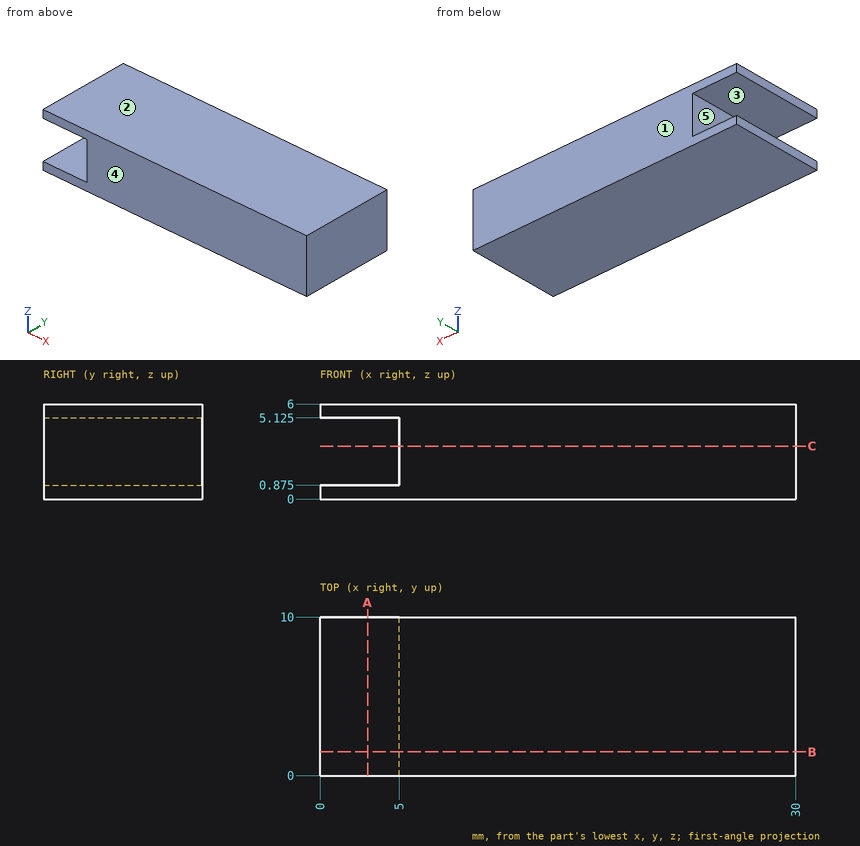
Answer from the drawing. Dimensions are ordinates in mm from the lowest x, y and z of the part. A direction names the side the tool comes from. Coordinates: 2 decimals unless noted, no trailing zeros. Order: outer loops, then holes, each group sorted by start corner. A loop starts at its lowest first (then second) coordinate and runs counter-clockwise, first axis right, second up. Notation, with made-up numbers: (-31.5, 34) - (-19.5, 34) arc R12 cw to (-19.5, 38) - close; hole circle Ø3 at (-14, 87). An arc over 180 degrees is marked (long way). Use one line per item in the form item = value.
(1) Which of the six approach directions +Z, -Z, +X, -X, +Y, -Y give full straight-line access (tool end or side, diameter ignored) to the marked faces 4 and 5?
Computed values:
face_4 = +Z, -Z, +X, -X, -Y
face_5 = -X, +Y, -Y
(2) Section A-A, the plane x = 3 is taken. Give the vertices of the cut face in (y, z) (3 decimals), then the cut area to 3 significant figures.
Computed values:
outline = (0, 0) - (10, 0) - (10, 0.875) - (0, 0.875) - close; (0, 5.125) - (10, 5.125) - (10, 6) - (0, 6) - close
area = 17.5 mm²
(3) Section B-B, the plane y = 1.5 is taken. Give the vertices of the cut face in (x, z) (3 decimals), then the cut area to 3 significant figures.
Computed values:
outline = (0, 0) - (30, 0) - (30, 6) - (0, 6) - (0, 5.125) - (5, 5.125) - (5, 0.875) - (0, 0.875) - close
area = 159 mm²
(4) Given pin 1 Ø3.5 at (y, z) = (4.5, 4) entering from -X, flat-ended and moving along its own axis, determine where the tip first touches the part or whether it passes through.
Computed values:
pin_1 = 0
(5) For a pull along Z with two mould halves and no side action, classify the marked faces 1, 2 and 3 as pulls with the +Z half, pulls with the -Z half, needs draft (parallel to the pull), parting line crosses it, or undercut.
Computed values:
face_1 = needs draft
face_2 = pulls with the +Z half
face_3 = undercut
(6) Section C-C, the plane z = 3.35 is taken. Give the vertices of the cut face in (x, y), then the cut area to 3 significant figures.
Computed values:
outline = (5, 0) - (30, 0) - (30, 10) - (5, 10) - close
area = 250 mm²
(7) Straight lines are drawn through the part: L1, parallel to Z at x = 2.75, y = 5 (3 decimals); L2, parallel to X at y = 5, z = 5. For each, find the intervals that lie inside material, in ascending order.
Computed values:
L1 = 0 to 0.875, 5.125 to 6
L2 = 5 to 30
